The model under review builds one solid part; all positions refer to its coordinate system, in mm. A direction names the side the tool comes from. Coordinates: 2 decimals unless noted, no trailing zeros. Loops run counter-clockwise (first coordinate to the right, second up) from the corner with the lowest first, then second, coordinate; pieces in that order, holes last. Notation, with made-up numbers: (59, 62.5) - (83, 62.5) arc R35 ccw to (83, 95.5) - close; hole circle Ø10 at (83, -16.75). An arc over 180 degrees is marked (long way). Use a Markdown table: item, result. Add a question column.
1) Clearance check with flat-ended pins moving along their axes: pin 1 (1.5 mm diameter, centred on x = 8.5, z = 0, fed in from +Y); pin 2 (5 mm diameter, centred on x = 9, z = -1.5, fed in from -Y); pin 3 (1 mm diameter, centred on y = 2, z = -3, fed in from +X); pin 4 (10 mm diameter, centred on x = -10.5, y = 13.5, fed in from -Z). State where each tip first meets the part, or that it passes through.
2) Add section B-B, the plane x = -1. Give the boundary of the cut face in (y, z).
3) The part is to be moulded in two halves that separate along X. For faces 1 (the flat face through (2.2, -7, 3.3)), 2 (the flat face through (12.5, 23, 0)), 3 (the flat face through (19.5, 12, 0)), say which applies: pulls with the +X half, pulls with the -X half, needs draft (parallel to the pull), parting line crosses it, or undercut.
4) Add section A-A, the plane y = 11. Give the boundary of the cut face in (x, z), and give its area (3 significant figures).
5) For faces 4 (the flat face through (-12.5, 23, 0)), 5 (the flat face through (17, 28, 0)), 6 (the flat face through (0, -5, 0)), list the 3-axis set-ups (+Z, -Z, +X, -X, +Y, -Y) from which the entire face can be reached by the end or side of a thin tool; tool diameter is ignored.
6) To check wall thickness, follow L1, parallel to X at y = 20, z = 1.5; L2, parallel to X at y = 9, z = -1; L3, parallel to Y at x = 17, z = -0.25. State the ranges of each line that lie inside material, in increasing order. Write a range as [from, to].
7) Add section D-D, the plane y = 22.5. Give the boundary of the cut face in (x, z), and give its area (3 significant figures).
8) Add section C-C, the plane z = 4.5. Give the boundary of the cut face in (x, y).
```python
from build123d import *

# Parameters (mm, degrees)
BOSS_EXTRU_2_DEPTH      = 5
BOSS_EXTRU_3_DEPTH      = 28
ESQUISSE3_R             = 3.5
BOSS_EXTRU_5_DEPTH      = 2
BOSS_EXTRU_5_DEPTH_BACK = 1
BOSS_EXTRU_7_DEPTH      = 7
ESQUISSE4_R             = 3.5
BOSS_EXTRU_8_DEPTH      = 2
BOSS_EXTRU_8_DEPTH_BACK = 1


with BuildPart() as part:
    # Esquisse1 → Boss.-Extru.2 (new body)
    with BuildSketch(Plane(origin=(0, 0, 0), x_dir=(1, 0, 0), z_dir=(0, 1, 0))):
        with BuildLine():
            Line((-17, -5), (17, -5))
            ThreePointArc((17, -5), (18.767766953, -4.267766953), (19.5, -2.5))
            Line((19.5, -2.5), (19.5, 2.5))
            ThreePointArc((19.5, 2.5), (18.767766953, 4.267766953), (17, 5))
            Line((17, 5), (-17, 5))
            ThreePointArc((-17, 5), (-18.767766953, 4.267766953), (-19.5, 2.5))
            Line((-19.5, 2.5), (-19.5, -2.5))
            ThreePointArc((-19.5, -2.5), (-18.767766953, -4.267766953), (-17, -5))
        make_face()
    extrude(amount=-BOSS_EXTRU_2_DEPTH)

    # Esquisse1<6> → Boss.-Extru.3 (add)
    with BuildSketch(Plane(origin=(0, 0, 0), x_dir=(1, 0, 0), z_dir=(0, 1, 0))):
        with BuildLine():
            ThreePointArc((-19.5, -2.5), (-17, -5), (-14.5, -2.5))
            Line((-14.5, -2.5), (-14.5, 2.5))
            ThreePointArc((-14.5, 2.5), (-17, 5), (-19.5, 2.5))
            Line((-19.5, 2.5), (-19.5, -2.5))
        make_face()
        with BuildLine():
            ThreePointArc((14.5, -2.5), (17, -5), (19.5, -2.5))
            Line((19.5, -2.5), (19.5, 2.5))
            ThreePointArc((19.5, 2.5), (17, 5), (14.5, 2.5))
            Line((14.5, 2.5), (14.5, -2.5))
        make_face()
    extrude(amount=BOSS_EXTRU_3_DEPTH)

    # Esquisse3 → Boss.-Extru.5 (add, two sides)
    with BuildSketch(Plane(origin=(-14.5, 0, 0), x_dir=(0, 0, -1), z_dir=(1, 0, 0))) as boss_extru_5_sk:
        with Locations((0, 23)):
            Circle(ESQUISSE3_R)
    extrude(amount=BOSS_EXTRU_5_DEPTH)
    extrude(boss_extru_5_sk.sketch, amount=-BOSS_EXTRU_5_DEPTH_BACK)

    # Esquisse1<9> → Boss.-Extru.7 (add)
    with BuildSketch(Plane(origin=(0, 0, 0), x_dir=(1, 0, 0), z_dir=(0, 1, 0))):
        with BuildLine():
            ThreePointArc((-5, 0), (-3.535533906, -3.535533906), (0, -5))
            ThreePointArc((0, -5), (3.535533906, -3.535533906), (5, 0))
            Line((5, 0), (3.5, 0))
            ThreePointArc((3.5, 0), (0, -3.5), (-3.5, 0))
            Line((-3.5, 0), (-5, 0))
        make_face()
        with BuildLine():
            Line((3.5, 0), (5, 0))
            ThreePointArc((5, 0), (3.535533906, 3.535533906), (0, 5))
            ThreePointArc((0, 5), (-3.535533906, 3.535533906), (-5, 0))
            Line((-5, 0), (-3.5, 0))
            ThreePointArc((-3.5, 0), (0, 3.5), (3.5, 0))
        make_face()
    extrude(amount=-BOSS_EXTRU_7_DEPTH)

    # Esquisse4 → Boss.-Extru.8 (add, two sides)
    with BuildSketch(Plane.ZY.offset(-14.5)) as boss_extru_8_sk:
        with Locations((0, 23)):
            Circle(ESQUISSE4_R)
    extrude(amount=BOSS_EXTRU_8_DEPTH)
    extrude(boss_extru_8_sk.sketch, amount=-BOSS_EXTRU_8_DEPTH_BACK)


solid = part.part
```
From the geometry:
| question | item | result |
|---|---|---|
| 1 | pin 1 | stops at y = 0 |
| 1 | pin 2 | stops at y = -5 |
| 1 | pin 3 | stops at x = 19.5 |
| 1 | pin 4 | stops at z = -4.5 |
| 2 | outline | (-7, -4.9) - (-5, -4.9) - (-5, -5) - (0, -5) - (0, 5) - (-5, 5) - (-5, 4.9) - (-7, 4.9) - (-7, 3.35) - (-5, 3.35) - (-5, -3.35) - (-7, -3.35) - close |
| 3 | face 1 | needs draft |
| 3 | face 2 | undercut |
| 3 | face 3 | pulls with the +X half |
| 4 | outline | (-19.5, -2.5) arc R2.5 ccw to (-14.5, -2.5) - (-14.5, 2.5) arc R2.5 ccw to (-19.5, 2.5) - close; (14.5, -2.5) arc R2.5 ccw to (19.5, -2.5) - (19.5, 2.5) arc R2.5 ccw to (14.5, 2.5) - close |
| 4 | area | 89.3 mm^2 |
| 5 | face 4 | +Z, -Z, +Y |
| 5 | face 5 | +Z, -Z, +X, -X, +Y |
| 5 | face 6 | -Y |
| 6 | L1 | x = [-19.5, -12.5], [12.5, 19.5] |
| 6 | L2 | x = [-19.5, -14.5], [14.5, 19.5] |
| 6 | L3 | y = [-5, 28] |
| 7 | outline | (-19.5, -2.5) arc R2.5 ccw to (-14.69, -3.46) - (-12.5, -3.46) - (-12.5, 3.46) - (-14.69, 3.46) arc R2.5 ccw to (-19.5, 2.5) - close; (12.5, -3.46) - (14.69, -3.46) arc R2.5 ccw to (19.5, -2.5) - (19.5, 2.5) arc R2.5 ccw to (14.69, 3.46) - (12.5, 3.46) - close |
| 7 | area | 117 mm^2 |
| 8 | outline | (-18.5, -5) - (-2.18, -5) - (-2.18, -7) - (2.18, -7) - (2.18, -5) - (18.5, -5) - (18.5, 28) - (15.5, 28) - (15.5, 0) - (-15.5, 0) - (-15.5, 28) - (-18.5, 28) - close |
